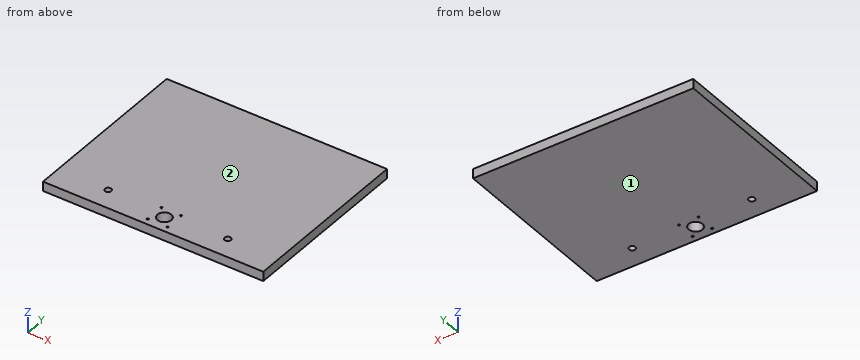
```python
from build123d import *

# Parameters (mm, degrees)
SKETCH3_W           = 350
SKETCH3_H           = 280
SKETCH3_R           = 1.5
SKETCH3_R_2         = 11
SKETCH3_R_3         = 5
BOSS_EXTRUDE3_DEPTH = 15


with BuildPart() as part:
    # Sketch3 → Boss-Extrude3 (new body)
    with BuildSketch(Plane.XY):
        with Locations((369.918861249, 211.697453917)):
            Rectangle(SKETCH3_W, SKETCH3_H)
        with Locations((354.418861249, 112.697453917)):
            Circle(SKETCH3_R, mode=Mode.SUBTRACT)
        with Locations((385.418861249, 112.697453917)):
            Circle(SKETCH3_R, mode=Mode.SUBTRACT)
        with Locations((354.418861249, 81.697453917)):
            Circle(SKETCH3_R, mode=Mode.SUBTRACT)
        with Locations((385.418861249, 81.697453917)):
            Circle(SKETCH3_R, mode=Mode.SUBTRACT)
        with Locations((369.918861249, 97.197453917)):
            Circle(SKETCH3_R_2, mode=Mode.SUBTRACT)
        with Locations((274.918861249, 105.197453917)):
            Circle(SKETCH3_R_3, mode=Mode.SUBTRACT)
        with Locations((464.918861249, 105.197453917)):
            Circle(SKETCH3_R_3, mode=Mode.SUBTRACT)
    extrude(amount=BOSS_EXTRUDE3_DEPTH)


solid = part.part
```
Part model, mm, in its own coordinate system. Face numbers are marked on the shaded views. Round coordinates to 2 decimals unless told otherwise and drop trailing zeros. Loops run counter-clockwise (first coordinate to the right, second up) from the corner with the lowest first, then second, coordinate; pieces in that order, holes last.
Item 1: Drill centre lines: line 1 (X direction, y = 96.5, z = 11.25); line 2 (X direction, y = 92, z = 9.5); line 3 (Y direction, x = 376.5, z = 5.75). Where is each one in solid material? Low to high.
Item 2: Mould opens along Z. For the marked faces 1 and 2 say: +Z half, -Z half, draft (parallel to the pull), parting line (faces both ways), or undercut.
Item 3: Cut at A-A, the plane x = 275.5. Give the cut face in (y, z).
A:
1. line 1: x = 194.92 to 358.94, 380.9 to 544.92
1. line 2: x = 194.92 to 360.22, 379.61 to 544.92
1. line 3: y = 71.7 to 88.38, 106.01 to 351.7
2. face 1: -Z half
2. face 2: +Z half
3. outline: (71.7, 0) - (100.23, 0) - (100.23, 15) - (71.7, 15) - close; (110.16, 0) - (351.7, 0) - (351.7, 15) - (110.16, 15) - close
